Geometry check sheet. Reference: the model listing, model coordinates, mm. A direction names the side the tool comes from. Round coordinates to 2 decimals unless told otherwise and drop trailing zeros. Loops run counter-clockwise (first coordinate to the right, second up) from the corner with the lowest first, then second, coordinate; pieces in that order, holes last.
```python
from build123d import *

# Parameters (mm, degrees)
SKETCH1_W           = 15
SKETCH1_H           = 60
BOSS_EXTRUDE1_DEPTH = 70
SKETCH2_R           = 17
CUT_EXTRUDE1_DEPTH  = 70
SKETCH3_W           = 60
SKETCH3_H           = 40
CUT_EXTRUDE2_DEPTH  = 29
SKETCH4_R           = 2
CUT_EXTRUDE3_DEPTH  = 6
SKETCH5_R           = 2
CUT_EXTRUDE4_DEPTH  = 10
SKETCH6_R           = 2
CUT_EXTRUDE5_DEPTH  = 14
CUT_EXTRUDE6_START  = -14
SKETCH7_R           = 2
CUT_EXTRUDE6_DEPTH  = 14


with BuildPart() as part:
    # Sketch1 → Boss-Extrude1 (new body)
    with BuildSketch(Plane(origin=(0, 0, 0), x_dir=(1, 0, 0), z_dir=(0, 1, 0))):
        Rectangle(SKETCH1_W, SKETCH1_H)
    extrude(amount=BOSS_EXTRUDE1_DEPTH)

    # Sketch2 → Cut-Extrude1 (cut)
    with BuildSketch(Plane(origin=(7.5, 0, 0), x_dir=(0, 0, -1), z_dir=(1, 0, 0))):
        with Locations((0, 30)):
            Circle(SKETCH2_R)
    extrude(amount=-CUT_EXTRUDE1_DEPTH, mode=Mode.SUBTRACT)

    # Sketch3 → Cut-Extrude2 (cut)
    with BuildSketch(Plane(origin=(7.5, 0, 0), x_dir=(0, 0, -1), z_dir=(1, 0, 0))):
        with Locations((0, 50)):
            Rectangle(SKETCH3_W, SKETCH3_H)
    extrude(amount=-CUT_EXTRUDE2_DEPTH, mode=Mode.SUBTRACT)

    # Sketch4 → Cut-Extrude3 (cut)
    with BuildSketch(Plane(origin=(0, 30, 0), x_dir=(1, 0, 0), z_dir=(0, 1, 0))):
        with Locations(Location((-4, 24, 0), (0, 0, 270))):
            Circle(SKETCH4_R)
        with Locations(Location((4, 24, 0), (0, 0, 270))):
            Circle(SKETCH4_R)
        with Locations(Location((-4, -24, 0), (0, 0, 270))):
            Circle(SKETCH4_R)
        with Locations(Location((4, -24, 0), (0, 0, 270))):
            Circle(SKETCH4_R)
    extrude(amount=-CUT_EXTRUDE3_DEPTH, mode=Mode.SUBTRACT)

    # Sketch5 → Cut-Extrude4 (cut)
    with BuildSketch(Plane(origin=(7.5, 0, 0), x_dir=(0, 0, -1), z_dir=(1, 0, 0))):
        with Locations((-16, 14)):
            Circle(SKETCH5_R)
        with Locations((16, 14)):
            Circle(SKETCH5_R)
    extrude(amount=-CUT_EXTRUDE4_DEPTH, mode=Mode.SUBTRACT)

    # Sketch6 → Cut-Extrude5 (cut)
    with BuildSketch(Plane(origin=(0, 0, -30), x_dir=(-1, 0, 0), z_dir=(0, 0, -1))):
        with Locations((0, 4)):
            Circle(SKETCH6_R)
    extrude(amount=-CUT_EXTRUDE5_DEPTH, mode=Mode.SUBTRACT)

    # Sketch7 → Cut-Extrude6 (cut)
    with BuildSketch(Plane.XY.offset(30).offset(CUT_EXTRUDE6_START)):
        with Locations(Location((0, 4, 0), (0, 0, 180))):
            Circle(SKETCH7_R)
    extrude(amount=CUT_EXTRUDE6_DEPTH, mode=Mode.SUBTRACT)


solid = part.part
```
1) Sectioned sample at B-B, the plane x = 0. Record the cut outline in (y, z), then the cut area to 3 significant figures.
Report:
outline: (0, -30) - (2, -30) - (2, -16) - (6, -16) - (6, -30) - (30, -30) - (30, -17) arc R17 cw to (30, 17) - (30, 30) - (6, 30) - (6, 16) - (2, 16) - (2, 30) - (0, 30) - close; hole circle Ø4 at (14, -16); hole circle Ø4 at (14, 16)
area: 1,210 mm2
2) Sectioned sample at D-D, the plane y = 4. Record the cut outline in (x, z).
Report:
outline: (-7.5, -30) - (-2, -30) - (-2, -16) - (2, -16) - (2, -30) - (7.5, -30) - (7.5, 30) - (2, 30) - (2, 16) - (-2, 16) - (-2, 30) - (-7.5, 30) - close
3) Sectioned sample at A-A, the plane z = 21. Record the cut outline in (x, y).
Report:
outline: (-7.5, 0) - (7.5, 0) - (7.5, 30) - (-7.5, 30) - close; hole circle Ø4 at (0, 4)
4) Scan lines: line 1 along X through (y, z) = (27.8, 24); line 2 along Z through (x, y) = (-3.5, 26.5); line 3 along Z through (x, y) = (0.5, 12.5). Record each from-to range of solid material in increasing order.
Report:
line 1: x = -7.5 to -6, -2 to 2, 6 to 7.5
line 2: z = -30 to -25.94, -22.06 to -16.64, 16.64 to 22.06, 25.94 to 30
line 3: z = -30 to -17.32, -14.68 to 14.68, 17.32 to 30
5) Mould release check, pull along X, two halves, no side actions. Record for faces 1 (the face through (7.5, 11, 0)), 2 (the face through (0, 15, -30)), 3 (the face through (4, 24, 24)), 4 (the face through (-5.2, 27, -25.6)): +X half, -X half, draft (parallel to the pull), parting line (faces both ways), or undercut.
Report:
face 1: +X half
face 2: draft
face 3: undercut
face 4: undercut
6) Sectioned sample at C-C, the plane y = 14. Record the cut outline in (x, z).
Report:
outline: (-7.5, -30) - (7.5, -30) - (7.5, -18) - (-2.5, -18) - (-2.5, -14) - (7.5, -14) - (7.5, -5.74) - (-7.5, -5.74) - close; (-7.5, 5.74) - (7.5, 5.74) - (7.5, 14) - (-2.5, 14) - (-2.5, 18) - (7.5, 18) - (7.5, 30) - (-7.5, 30) - close
7) Access from +Z, -Z, +X, -X, +Y, -Y to the whole of each face (thin tool, end or side, straight path). Record for faces 5 (the face through (-2.5, 14, -16)), 6 (the face through (2.8, 27, 22.4)), 7 (the face through (0, 2, -23)).
Report:
face 5: +X
face 6: +Y
face 7: -Z
8) Gauge pin test, flat ends, axial feed: pin 1 (2 mm diameter, centred on x = -3.5, z = 23.5, fed in from +Y); pin 2 (1 mm diameter, centred on x = 1, z = 5, fed in from +Y); pin 3 (1.2 mm diameter, centred on y = 14, z = -16, fed in from +X). Record the tip position at first contact, or that the pin passes through.
Report:
pin 1: stops at y = 24
pin 2: stops at y = 13.91
pin 3: stops at x = -2.5
